```python
from build123d import *

# Parameters (mm, degrees)
BODY_DEPTH  = 1.0668
HOLSKE_R    = 0.9906
HOLES_DEPTH = 2.0668


with BuildPart() as part:
    # BodySke → Body (new body)
    with BuildSketch(Plane.XY):
        with BuildLine():
            Line((0.754834919, -4.676573602), (1.325514402, -8.212213698))
            Line((1.325514402, -8.212213698), (2.830042103, -7.969371365))
            ThreePointArc((2.830042103, -7.969371365), (3.988232781, -7.254926373), (4.302008364, -5.930772992))
            Line((4.302008364, -5.930772992), (4.202374684, -5.313493335))
            ThreePointArc((4.202374684, -5.313493335), (4.246706733, -4.824497903), (4.520407312, -4.416858533))
            ThreePointArc((4.520407312, -4.416858533), (0, 7.4295), (-4.520407312, -4.416858533))
            ThreePointArc((-4.520407312, -4.416858533), (-4.246706733, -4.824497903), (-4.202374684, -5.313493335))
            Line((-4.202374684, -5.313493335), (-4.302008364, -5.930772992))
            ThreePointArc((-4.302008364, -5.930772992), (-3.988232781, -7.254926373), (-2.830042103, -7.969371365))
            Line((-2.830042103, -7.969371365), (-1.325514402, -8.212213698))
            Line((-1.325514402, -8.212213698), (-0.754834919, -4.676573602))
            ThreePointArc((-0.754834919, -4.676573602), (0, 4.7371), (0.754834919, -4.676573602))
        make_face()
    extrude(amount=-BODY_DEPTH)

    # HolSke → Holes (cut, through all)
    with BuildSketch(Plane.XY):
        with Locations((2.546726047, -6.214089047)):
            Circle(HOLSKE_R)
        with Locations((-2.546726047, -6.214089047)):
            Circle(HOLSKE_R)
    extrude(amount=-HOLES_DEPTH, mode=Mode.SUBTRACT)


solid = part.part
```
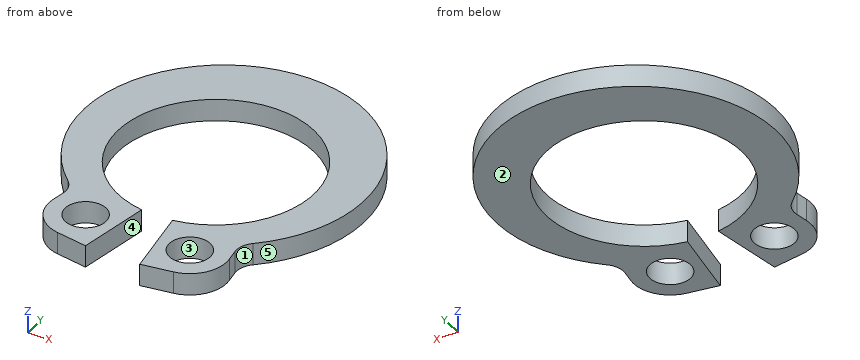
Can you work these out from the model? Positions are in its coordinate system, mm. Face numbers are marked on the shaded views. A direction names the side the tool comes from. Give positions to 0.01 mm unless a question says otherwise; leave off trailing zeros. Loops run counter-clockwise (first coordinate to the right, second up) from the corner with the lowest first, then second, coordinate; pieces in that order, holes last. Notation, with made-up numbers: M 58.5,50 L 98.5,50 A24 cw 98.5,70 Z; hole C 4,51 d5. An arc over 180 degrees is marked long. Use one line per item in the form item = value. Start each with the question number.
(1) Please list where these lines run through material, in increasing order: line 1 (Y direction, x = -2.5, z = -0.25); line 2 (Y direction, x = -2.25, z = -0.05); line 3 (Y direction, x = 0, z = -0.4).
(2) I'm going to push a flat-ended pin straight in: P1, Ø1, axis at x = 0, y = 3.5, coming from the +Z side. Where does the tip first touch, or does it pass through?
(3) On a 3-axis mill with a long thin cutter (end or side, diameter ignored), from which of +Z, -Z, +X, -X, +Y, -Y can I reach the whole of each face in a straight line? I mean the marked faces 4 and 5. Say none if no direction works.
(4) I want a section at D-D, the plane z = -0.25. Write out the boundary of the cut face in (x, y), and give its area (3 significant figures).
(5) I want a section at C-C, the plane y = -7. Write out the boundary of the cut face in (x, z), and give its area (3 significant figures).
(6) I want a section at A-A, the plane y = -0.25. Write out the boundary of the cut face in (x, z), and give its area (3 significant figures).
(7) I want a section at B-B, the plane x = -3.25. Write out the boundary of the cut face in (y, z).
(8) Thinking about a two-plate mould opening in X: for the marked faces 1, 2 and 3, which applies, released by +X, released by -X, zero draft, split by the parting line, or undercut?
Worked out:
q1.line_1 = -8.02 to -7.2, -5.22 to -4.02, 4.02 to 6.95
q1.line_2 = -8.06 to -7.16, -5.27 to -4.17, 4.17 to 7.05
q1.line_3 = 4.74 to 7.43
q2.P1 = through
q3.face_4 = +Z, -Z, -Y
q3.face_5 = +Z, -Z
q4.outline = M -4.52,-4.42 A0.99 cw -4.2,-5.31 L -4.3,-5.93 A1.78 ccw -2.83,-7.97 L -1.33,-8.21 L -0.75,-4.68 A4.74 cw long 0.75,-4.68 L 1.33,-8.21 L 2.83,-7.97 A1.78 ccw 4.3,-5.93 L 4.2,-5.31 A0.99 cw 4.52,-4.42 A6.79 ccw long Z; hole C -2.55,-6.21 d1.98; hole C 2.55,-6.21 d1.98
q4.area = 80.3 mm²
q5.outline = M -4.14,-1.07 L -3.15,-1.07 L -3.15,0 L -4.14,0 Z; M -1.94,-1.07 L -1.13,-1.07 L -1.13,0 L -1.94,0 Z; M 1.13,-1.07 L 1.94,-1.07 L 1.94,0 L 1.13,0 Z; M 3.15,-1.07 L 4.14,-1.07 L 4.14,0 L 3.15,0 Z
q5.area = 3.85 mm²
q6.outline = M -6.73,-1.07 L -4.73,-1.07 L -4.73,0 L -6.73,0 Z; M 4.73,-1.07 L 6.73,-1.07 L 6.73,0 L 4.73,0 Z
q6.area = 4.26 mm²
q7.outline = M -7.85,-1.07 L -6.91,-1.07 L -6.91,0 L -7.85,0 Z; M -5.52,-1.07 L -3.45,-1.07 L -3.45,0 L -5.52,0 Z; M 3.45,-1.07 L 6.6,-1.07 L 6.6,0 L 3.45,0 Z
q8.face_1 = released by +X
q8.face_2 = zero draft
q8.face_3 = undercut
